from build123d import *

# Parameters (mm, degrees)
SKETCH1_W               = 1922.702167778
SKETCH1_H               = 1506.854577214
BOSS_EXTRUDE1_DEPTH     = 20
SKETCH2_R               = 20.121201263
CUT_EXTRUDE1_DEPTH      = 20
CUT_EXTRUDE2_DEPTH      = 1222.576270935
CUT_EXTRUDE3_DEPTH      = 1222.576270935
CUT_EXTRUDE4_DEPTH      = 1222.576270935
CUT_EXTRUDE4_DEPTH_BACK = 1222.576270935
CUT_EXTRUDE5_DEPTH      = 1222.576270935
CUT_EXTRUDE6_DEPTH      = 1222.576270935


with BuildPart() as part:
    # Sketch1 → Boss-Extrude1 (new body)
    with BuildSketch(Plane(origin=(0, 0, 0), x_dir=(1, 0, 0), z_dir=(0, 1, 0))):
        Rectangle(SKETCH1_W, SKETCH1_H)
    extrude(amount=BOSS_EXTRUDE1_DEPTH)

    # Sketch2 → Cut-Extrude1 (cut)
    with BuildSketch(Plane(origin=(0, 20, 0), x_dir=(1, 0, 0), z_dir=(0, 1, 0))):
        with Locations(Location((0, 0, 0), (0, 0, 270))):
            Circle(SKETCH2_R)
    extrude(amount=-CUT_EXTRUDE1_DEPTH, mode=Mode.SUBTRACT)

    # Sketch3 → Cut-Extrude2 (cut, through all)
    with BuildSketch(Plane(origin=(0, 20, 0), x_dir=(1, 0, 0), z_dir=(0, 1, 0))):
        with BuildLine():
            Line((-501.853893247, 28.082670062), (-351.853893247, 28.082670062))
            ThreePointArc((-351.853893247, 28.082670062), (-323.771223185, 0), (-351.853893247, -28.082670062))
            Line((-351.853893247, -28.082670062), (-501.853893247, -28.082670062))
            ThreePointArc((-501.853893247, -28.082670062), (-529.936563308, 0), (-501.853893247, 28.082670062))
        make_face()
    extrude(amount=-CUT_EXTRUDE2_DEPTH, mode=Mode.SUBTRACT)

    # Sketch4 → Cut-Extrude3 (cut, through all)
    with BuildSketch(Plane(origin=(0, 20, 0), x_dir=(1, 0, 0), z_dir=(0, 1, 0))):
        with BuildLine():
            Line((530.111507452, 3.430580165), (620.111507452, 3.430580165))
            ThreePointArc((620.111507452, 3.430580165), (634.253643076, 9.288444541), (640.111507452, 23.430580165))
            Line((640.111507452, 23.430580165), (640.111507452, 98.430580165))
            ThreePointArc((640.111507452, 98.430580165), (634.253643076, 112.572715788), (620.111507452, 118.430580165))
            Line((620.111507452, 118.430580165), (530.111507452, 118.430580165))
            ThreePointArc((530.111507452, 118.430580165), (515.969371828, 112.572715788), (510.111507452, 98.430580165))
            Line((510.111507452, 98.430580165), (510.111507452, 23.430580165))
            ThreePointArc((510.111507452, 23.430580165), (515.969371828, 9.288444541), (530.111507452, 3.430580165))
        make_face()
    extrude(amount=-CUT_EXTRUDE3_DEPTH, mode=Mode.SUBTRACT)

    # Sketch5 → Cut-Extrude4 (cut, two sides: drawn at the far end of the back side and taken through both)
    with BuildSketch(Plane(origin=(0, 20, 0), x_dir=(1, 0, 0), z_dir=(0, 1, 0)).offset(-CUT_EXTRUDE4_DEPTH_BACK)):
        with BuildLine():
            Line((-182.264012939, 403.894827106), (-112.264012939, 403.894827106))
            ThreePointArc((-112.264012939, 403.894827106), (-91.050809503, 412.681623671), (-82.264012939, 433.894827106))
            Line((-82.264012939, 433.894827106), (-82.264012939, 488.894827106))
            ThreePointArc((-82.264012939, 488.894827106), (-91.050809503, 510.108030542), (-112.264012939, 518.894827106))
            Line((-112.264012939, 518.894827106), (-182.264012939, 518.894827106))
            ThreePointArc((-182.264012939, 518.894827106), (-203.477216375, 510.108030542), (-212.264012939, 488.894827106))
            Line((-212.264012939, 488.894827106), (-212.264012939, 433.894827106))
            ThreePointArc((-212.264012939, 433.894827106), (-203.477216375, 412.681623671), (-182.264012939, 403.894827106))
        make_face()
    extrude(amount=CUT_EXTRUDE4_DEPTH + CUT_EXTRUDE4_DEPTH_BACK, mode=Mode.SUBTRACT)

    # Sketch6 → Cut-Extrude5 (cut, through all)
    with BuildSketch(Plane(origin=(0, 20, 0), x_dir=(1, 0, 0), z_dir=(0, 1, 0))):
        with BuildLine():
            Line((-803.044857879, 518.477090235), (-768.447719913, 553.074228201))
            ThreePointArc((-768.447719913, 553.074228201), (-759.794991438, 558.855796528), (-749.588402288, 560.886013339))
            Line((-749.588402288, 560.886013339), (-622.318858343, 560.886013339))
            ThreePointArc((-622.318858343, 560.886013339), (-595.647755579, 534.214910576), (-622.318858343, 507.543807813))
            Line((-622.318858343, 507.543807813), (-738.5408698, 507.543807813))
            Line((-738.5408698, 507.543807813), (-765.326222628, 480.758454984))
            ThreePointArc((-765.326222628, 480.758454984), (-803.044857879, 480.758454984), (-803.044857879, 518.477090235))
        make_face()
    extrude(amount=-CUT_EXTRUDE5_DEPTH, mode=Mode.SUBTRACT)

    # Sketch8 → Cut-Extrude6 (cut, through all)
    with BuildSketch(Plane(origin=(0, 20, 0), x_dir=(1, 0, 0), z_dir=(0, 1, 0))):
        with BuildLine():
            Line((-730.19585764, -555.467097942), (-730.19585764, -537.888913931))
            ThreePointArc((-730.19585764, -537.888913931), (-717.979020313, -525.672076605), (-705.762182987, -537.888913931))
            Line((-705.762182987, -537.888913931), (-705.762182987, -555.467097942))
            ThreePointArc((-705.762182987, -555.467097942), (-717.979020313, -615.594356546), (-730.19585764, -555.467097942))
        make_face()
    extrude(amount=-CUT_EXTRUDE6_DEPTH, mode=Mode.SUBTRACT)


solid = part.part
Geometry check sheet. Reference: the model listing, model coordinates, mm. Coordinates: 2 decimals unless noted, no trailing zeros. Loops run counter-clockwise (first coordinate to the right, second up) from the corner with the lowest first, then second, coordinate; pieces in that order, holes last. Notation, with made-up numbers: (-20.5, -1.75) - (1.5, -1.75) arc R8 cw to (1.5, 6.25) - close; hole circle Ø1 at (3.25, 3.5). An arc over 180 degrees is marked (long way). Use one line per item in the form item = value. Start each with the question number.
Item 1: Thickness scan on probe 1 along X at (y, z) = (6.5, 0); probe 2 along X at (y, z) = (16.25, -480.5); probe 3 along Z at (x, y) = (568, 1.5). Record the ranges inside material, lowest first.
Item 2: Section check B-B, the plane y = 11.5. Give the number of separate pieces and of enclosed holes in the cut face, and give its area (3 significant figures).
Item 3: Mould release check, pull along X, two halves, no side actions. Record for faces 1 (the face through (-13, 0, 157)), 2 (the face through (-716.78, 10.14, 615.57)): +X half, -X half, draft (parallel to the pull), parting line (faces both ways), or undercut.
Item 4: Section check A-A, the plane x = 0. Enter the section's corners in (y, z), and give its area (3 significant figures).
Computed:
q1.probe_1 = -961.35 to -529.94, -323.77 to -20.12, 20.12 to 961.35
q1.probe_2 = -961.35 to -802.78, -765.59 to -212.26, -82.26 to 961.35
q1.probe_3 = -753.43 to -118.43, -3.43 to 753.43
q2.separate_pieces = 1
q2.enclosed_holes = 6
q2.area = 2,840,000 mm2
q3.face_1 = draft
q3.face_2 = undercut
q4.outline = (0, -753.43) - (20, -753.43) - (20, -20.12) - (0, -20.12) - close; (0, 20.12) - (20, 20.12) - (20, 753.43) - (0, 753.43) - close
q4.area = 29,300 mm2
